Could you check a few things on this model? Use its own coordinates, in mm. Face numbers are marked on the shaded views. A direction names the side the tool comes from. Coordinates: 2 decimals unless noted, no trailing zeros. Order: outer loops, then holes, each group sorted by start corner. A loop starts at its lowest first (then second) coordinate and runs counter-clockwise, first axis right, second up. Notation, with made-up numbers: (56.5, 2.5) - (64.5, 2.5) arc R7 cw to (64.5, 10.5) - close; hole circle Ø8 at (46, -39.5). An arc over 180 degrees is marked (long way). One line per item, written item: value.
Autodesk Inventor part; units mm, degrees
ref_plane "YZ Plane" through (0, 0, 0) normal (1, 0, 0) x (0, 1, 0)
ref_plane "XZ Plane" through (0, 0, 0) normal (0, 1, 0) x (-1, 0, 0)
ref_plane "XY Plane" through (0, 0, 0) normal (0, 0, 1) x (1, 0, 0)
sketch "Sketch1" plane through (0, 0, 0) normal (0, 1, 0) x (-1, 0, 0)
  line L0 (56.9199, 1.0144) -> (62.116, 4.0144)
  line L1 (62.116, 4.0144) -> (50, 25)
  line L2 (-50, 25) -> (-61.25, 5.5144)
  line L3 (0.7428, 5.2971) -> (50, 25)
  line L4 (-0.7428, 5.2971) -> (-50, 25)
  line L5 (42.5883, 14.6502) -> (56.9199, 1.0144)
  line L6 (-0.7428, 5.2971) -> (0, 5)
  line L7 (0.7428, 5.2971) -> (0, 5)
  circle A0 centre (47.5441, 18.66) radius 1.4
  circle A1 centre (55.9574, 8.1656) radius 1.4
  circle A2 centre (-55.9574, 8.1656) radius 1.4
  circle A3 centre (-47.5441, 18.66) radius 1.4
  line L8 (-39.2213, 15.6885) -> (0, 0)
  line L9 (42.5883, 14.6502) -> (40.8234, 16.3294)
  line L10 (40.8234, 16.3294) -> (0, 0)
  line L11 (-61.25, 5.5144) -> (-49.134, -1.4808)
  line L12 (-49.134, -1.4808) -> (-39.2213, 15.6885)
  point P0 (0, 0)
  dimension "d0" = 2.8
  dimension "d1" = 2.8
  dimension "d2" = 2.8
  dimension "d3" = 2.8
  dimension "d14" = 5
extrude "Extrusion1" add sketch "Sketch1" along normal blind 50
sketch "Sketch2" plane through (0, 50, 0) normal (0, 1, 0) x (1, 0, 0)
  circle A0 centre (47.5441, -18.66) radius 1.4
  circle A1 centre (55.9574, -8.1656) radius 1.4
  circle A2 centre (-55.9574, -8.1656) radius 1.4
  circle A3 centre (-47.5441, -18.66) radius 1.4
  line L0 (-40.8234, -16.3294) -> (-56.9199, -1.0144)
  line L1 (-56.9199, -1.0144) -> (-62.116, -4.0144)
  line L2 (-62.116, -4.0144) -> (-50, -25)
  line L3 (-50, -25) -> (0, -5)
  line L4 (0, -5) -> (50, -25)
  line L5 (50, -25) -> (61.25, -5.5144)
  line L6 (39.2213, -15.6885) -> (0, 0)
  line L7 (0, 0) -> (-40.8234, -16.3294)
  line L8 (61.25, -5.5144) -> (49.134, 1.4808)
  line L9 (49.134, 1.4808) -> (39.2213, -15.6885)
  point P0 (0, 0)
extrude "Extrusion2" add sketch "Sketch2" against normal blind 40 contours A0 | A1 | A2 | A3
sketch "Sketch3" plane through (0, 50, 0) normal (0, 1, 0) x (1, 0, 0)
  line L0 (-62.116, -4.0144) -> (-58.116, -4.0144) construction
  circle A0 centre (-57.3863, -6.5497) radius 1.4
  line L1 (61.25, -5.5144) -> (57.25, -5.5144) construction
  circle A1 centre (57.3863, -6.5497) radius 1.4
  circle A2 centre (57.3863, -6.5497) radius 2.75
  circle A3 centre (-57.3863, -6.5497) radius 2.75
  point P0 (0, 0)
  dimension "d10" = 2.8
  dimension "d15" = 2.8
  dimension "d16" = 5.5
  dimension "d17" = 5.5
extrude "Extrusion3" add sketch "Sketch3" along normal blind 30
fillet "Fillet1" radius 20 1 edges at (0, 25, 5)
properties part number "Front Support" material "ABS Plastic"
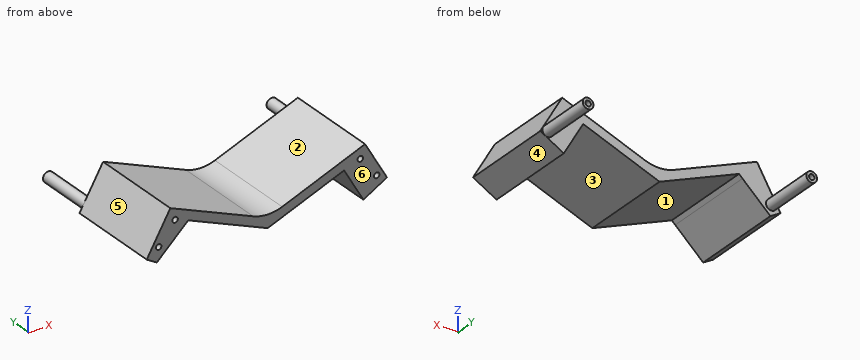
Item 1: If I drill on probe 1 along Y at (x, z) = (-28, 11.25); probe 2 along X at (y, z) = (15, 23.25) (3 decimals); probe 3 along X at (y, z) = (38.5, 22.75) (3 decimals), over which ranges is the centre line in solid material (lowest first)?
Conclusion:
probe 1: 0 to 50
probe 2: -51.01 to -45.625, 45.625 to 51.01
probe 3: -51.299 to -44.375, 44.375 to 51.299
Item 2: Thinking about a two-plate mould opening in X: for the marked faces 3, 4, 5 and 6, which applies, pulls with the +X half, pulls with the -X half, needs draft (parallel to the pull), parting line crosses it, or undercut?
Conclusion:
face 3: undercut
face 4: pulls with the +X half
face 5: pulls with the -X half
face 6: needs draft
Item 3: For the marked faces 1 and 2, which set-ups out of +Z, -Z, +X, -X, +Y, -Y let a thin tool reach every point of the face, with its end or its side?
Conclusion:
face 1: -Z, +Y, -Y
face 2: +Z, +Y, -Y
Item 4: I want a section at C-C on x = 14. Please give me the cut outline in (y, z), then the cut area to 3 significant figures.
Conclusion:
outline: (0, 5.6) - (50, 5.6) - (50, 10.6) - (0, 10.6) - close
area: 250 mm²
Item 5: I want a section at A-A on z = 18.66. Please give me the cut outline in (x, y).
Conclusion:
outline: (-53.66, 0) - (-48.94, 0) - (-48.94, 10) - (-46.14, 10) - (-46.14, 0) - (-34.15, 0) - (-34.15, 50) - (-53.66, 50) - close; (34.15, 0) - (46.14, 0) - (46.14, 10) - (48.94, 10) - (48.94, 0) - (53.66, 0) - (53.66, 50) - (34.15, 50) - close
Item 6: I want a section at B-B on y = 74. Please give me the cut outline in (x, z), then the cut area to 3 significant figures.
Conclusion:
outline: circle Ø5.5 at (-57.39, 6.55); circle Ø5.5 at (57.39, 6.55); hole circle Ø2.8 at (-57.39, 6.55); hole circle Ø2.8 at (57.39, 6.55)
area: 35.2 mm²
Item 7: I'm going to push flat-ended pins straight in: pin 1 Ø12 at (x, z) = (9.5, 17.5) entering from +Y; pin 2 Ø1.5 at (y, z) = (44.5, 20) entering from -X; pin 3 Ø2 at (x, y) = (-33.5, 48.5) entering from -Z; pin 4 Ø2.5 at (x, z) = (-47.54, 18.66) entering from +Y. Where does each tip first touch, or does it pass through?
Conclusion:
pin 1: through
pin 2: x = -53.32
pin 3: z = 13
pin 4: y = 50
